Autodesk Inventor part; units mm, degrees
ref_plane "YZ Plane" through (0, 0, 0) normal (1, 0, 0) x (0, 1, 0)
ref_plane "XZ Plane" through (0, 0, 0) normal (0, 1, 0) x (-1, 0, 0)
ref_plane "XY Plane" through (0, 0, 0) normal (0, 0, 1) x (1, 0, 0)
sketch "Эскиз1" plane through (0, 0, 0) normal (0, 0, 1) x (1, 0, 0)
  arc A0 (3.8683, 1.1995) -> (3.8683, -1.1995) centre (0, 0) ccw
  circle A1 centre (14, 0) radius 1.6
  line L0 (-17.8, 0) -> (50.8, 0) construction
  circle A2 centre (0, 0) radius 8
  circle A3 centre (35, 0) radius 6
  circle A4 centre (35, 0) radius 2.1
  line L1 (0.4571, 7.9869) -> (35.3429, 5.9902)
  line L2 (0.4571, -7.9869) -> (35.3429, -5.9902)
  circle A5 centre (19, 0) radius 1.6
  circle A6 centre (24, 0) radius 1.6
  circle A7 centre (29, 0) radius 1.6
  arc A8 (4.3318, -0.695) -> (4.3318, 0.695) centre (4.05, 0) ccw
  arc A9 (4.05, 0) -> (3.8683, 1.1995) centre (0, 0) ccw construction
  arc A10 (3.8683, -1.1995) -> (4.05, 0) centre (0, 0) ccw construction
  arc A11 (3.8683, 1.1995) -> (4.3318, 0.695) centre (4.6324, 1.4364) ccw
  arc A12 (4.3318, -0.695) -> (3.8683, -1.1995) centre (4.6324, -1.4364) ccw
  dimension "d0" = 8.1
  dimension "d1" = 3.2
  dimension "d2" = 14
  dimension "d3" = 16
  dimension "d5" = 12
  dimension "d6" = 35
  dimension "d7" = 4.2
  dimension "d22" = 5
  dimension "d27" = 1.5
  dimension "d28" = 0.8
extrude "Выдавливание1" add sketch "Эскиз1" along normal blind 6 contours A2 | A2 L1 A3 A7 L2 | A3 A7 picked at (31.3752, 2.1355)
chamfer "Фаска1" distance 0.6 angle 45 22 edges at (17.9, -6.9886, 0) (41, 0, 0) (17.9, 6.9886, 0) (-8, 0, 0) (12.4, 0, 0) (32.9, 0, 0) (17.9, 6.9886, 6) (-8, 0, 6) (17.9, -6.9886, 6) (41, 0, 6) (12.4, 0, 6) (32.9, 0, 6) (17.4, 0, 6) (22.4, 0, 6) (27.4, 0, 6) (27.4, 0, 0) (22.4, 0, 0) (17.4, 0, 0) (-4.05, 0, 0) (4.0433, 0.8951, 0) (4.8, 0, 0) (4.0433, -0.8951, 0)
properties part number "Рычаг натяжителя"
CAD build for the part. Positions are in the model's coordinates, mm. Round coordinates to 2 decimals unless told otherwise and drop trailing zeros. Loops run counter-clockwise (first coordinate to the right, second up) from the corner with the lowest first, then second, coordinate; pieces in that order, holes last. Notation, with made-up numbers: M -36.75,9.25 L 3.25,9.25 A16 cw 3.25,38.25 Z; hole C -7.5,55.5 d8. An arc over 180 degrees is marked long. Use a Markdown table: item, result. Add a question column.
(1) Flat gauge pins, fed straight in: pin 1 (3 mm diameter, centred on x = 24, y = 0, fed in from -Z); pin 2 (4 mm diameter, centred on x = 17, y = 6.5, fed in from -Z); pin 3 (1 mm diameter, centred on x = 4.5, z = 4, fed in from -Y); pin 4 (2 mm diameter, centred on y = 5, z = 0.5, fed in from +X). Where does each tip first touch, or does it go through?
(2) Drill centre lines: line 1 (Y direction, x = 24, z = 2.05); line 2 (Y direction, x = 14, z = 3.65); line 3 (Y direction, x = 39, z = 4.75). Where is each one in solid material? Low to high.
(3) Cut at A-A (x = 0). Give the cut face in (y, z).
(4) Cut at D-D (x = 14). Give the cut face in (y, z).
(5) Pull direction X, two halves, no side cores. Call faces 1 (the face through (16, -2, 6)), 2 (the face through (18.127, 6.671, 0.296)), 3 (the face through (4.8, 0, 3.3)): +X half, -X half, draft (parallel to the pull), parting line (faces both ways), or undercut.
(6) Cut at B-B (y = 0). State how many separate pieces and enclosed holes the cut face has, and give its area (3 significant figures).
Geometry says:
| question | item | result |
|---|---|---|
| 1 | pin 1 | passes through |
| 1 | pin 2 | stops at z = 0 |
| 1 | pin 3 | stops at y = -7.78 |
| 1 | pin 4 | stops at x = 39.47 |
| 2 | line 1 | y = -6.64 to -1.6, 1.6 to 6.64 |
| 2 | line 2 | y = -7.21 to -1.6, 1.6 to 7.21 |
| 2 | line 3 | y = -4.47 to 4.47 |
| 3 | outline | M -8,0.6 L -7.4,0 L -4.65,0 L -4.05,0.6 L -4.05,6 L -7.4,6 L -8,5.4 Z; M 4.05,0.6 L 4.65,0 L 7.4,0 L 8,0.6 L 8,5.4 L 7.4,6 L 4.05,6 Z |
| 4 | outline | M -7.21,0.6 L -6.61,0 L -2.2,0 L -1.6,0.6 L -1.6,5.4 L -2.2,6 L -6.61,6 L -7.21,5.4 Z; M 1.6,0.6 L 2.2,0 L 6.61,0 L 7.21,0.6 L 7.21,5.4 L 6.61,6 L 2.2,6 L 1.6,5.4 Z |
| 5 | face 1 | draft |
| 5 | face 2 | +X half |
| 5 | face 3 | undercut |
| 6 | separate pieces | 7 |
| 6 | enclosed holes | 0 |
| 6 | area | 134 mm² |
